Design review of the part built by this model. Coordinates are the model's own, in mm. A direction names the side the tool comes from. Coordinates: 2 decimals unless noted, no trailing zeros. Loops run counter-clockwise (first coordinate to the right, second up) from the corner with the lowest first, then second, coordinate; pieces in that order, holes last. Notation, with made-up numbers: (0.25, 78) -> (4.25, 78) arc R31 cw to (4.25, 107) -> close; hole circle Ø2 at (-9, 16). An arc over 180 degrees is marked (long way). Use a Markdown table: item, result. Add a question column.
Q1. For faces 1 (the face through (5, 10, 0)), 2 (the face through (12, 2, 0)), 3 (the face through (3, 0, 0)), list the 3-axis set-ups (+Z, -Z, +X, -X, +Y, -Y) from which the entire face can be reached by the end or side of a thin tool; tool diameter is ignored.
Q2. Take a section at A-A on y = 3.75. Write out the cut boundary in (x, z).
Q3. Clearance check with flat-ended pins moving along their axes: pin 1 Ø1.5 at (y, z) = (3, -4) entering from +X; pin 2 Ø5 at (y, z) = (10, 3.5) entering from +X; pin 3 Ø6 at (x, z) = (10, -0.5) entering from +Y. State where each tip first meets the part, or that it passes through.
Q4. Take a section at D-D on y = 10.5. Write out the cut boundary in (x, z), plus the area to 3 significant figures.
Q5. Take a section at C-C on x = 3.5. Write out the cut boundary in (y, z), plus the area to 4 significant figures.
Q6. For probe 1 along X at (y, z) = (4, -4.25); probe 2 along X at (y, z) = (7, 1.25); probe 3 along Y at (x, z) = (6, 8.25), list the stretches that pass through material, from the lowest coordinate up.
Q7. Take a section at B-B on z = -3. Write out the cut boundary in (x, y), plus the area to 3 significant figures.
from build123d import *

# Parameters (mm, degrees)
EXTRUDE_1_DEPTH     = 5
SKETCH_1_3_W        = 10
SKETCH_1_3_H        = 15
SKETCH_1_3_H_2      = 5
EXTRUDE_2_DEPTH     = 15
CUT_EXTRUDE_1_DEPTH = 15


with BuildPart() as part:
    # Sketch 1 → Extrude 1 (new body)
    with BuildSketch(Plane(origin=(0, 0, 0), x_dir=(1, 0, 0), z_dir=(0, 1, 0))):
        with BuildLine():
            ThreePointArc((15, -5), (13.535533906, -8.535533906), (10, -10))
            Line((10, -10), (5, -10))
            Line((5, -10), (5, 10))
            Line((5, 10), (10, 10))
            Line((10, 10), (10, 0))
            Line((10, 0), (15, 0))
            Line((15, 0), (15, -5))
        make_face()
    extrude(amount=EXTRUDE_1_DEPTH)

    # Sketch 1_3 → Extrude 2 (add)
    with BuildSketch(Plane(origin=(0, 0, 0), x_dir=(1, 0, 0), z_dir=(0, 1, 0))):
        with Locations((0, 2.5)):
            Rectangle(SKETCH_1_3_W, SKETCH_1_3_H)
        with Locations((0, -7.5)):
            Rectangle(SKETCH_1_3_W, SKETCH_1_3_H_2)
    extrude(amount=EXTRUDE_2_DEPTH)

    # Sketch 2 → Cut-Extrude 1 (cut)
    with BuildSketch(Plane.ZY.offset(5)):
        Polygon((5, 15), (10, 10), (10, 15), align=None)
    extrude(amount=-CUT_EXTRUDE_1_DEPTH, mode=Mode.SUBTRACT)


solid = part.part
Answer list:
| question | item | result |
|---|---|---|
| 1 | face 1 | +Z, -Z, +X, +Y |
| 1 | face 2 | -Z, +X, +Y, -Y |
| 1 | face 3 | +Z, -Z, +X, -X, -Y |
| 2 | outline | (-5, -10) -> (10, -10) -> (10, 0) -> (15, 0) -> (15, 5) arc R5 ccw to (10, 10) -> (-5, 10) -> close |
| 3 | pin 1 | x = 10 |
| 3 | pin 2 | x = 5 |
| 3 | pin 3 | y = 5 |
| 4 | outline | (-5, -10) -> (5, -10) -> (5, 9.5) -> (-5, 9.5) -> close |
| 4 | area | 195 mm² |
| 5 | outline | (0, -10) -> (15, -10) -> (15, 5) -> (10, 10) -> (0, 10) -> close |
| 5 | area | 287.5 mm² |
| 6 | probe 1 | -5 to 10 |
| 6 | probe 2 | -5 to 5 |
| 6 | probe 3 | 0 to 5 |
| 7 | outline | (-5, 0) -> (10, 0) -> (10, 5) -> (5, 5) -> (5, 15) -> (-5, 15) -> close |
| 7 | area | 175 mm² |
